For this review, take the finished solid that the model builds, in its own axes (mm). A direction names the side the tool comes from. Give positions to 0.01 mm unless a question says otherwise; leave off trailing zeros. Order: outer loops, then holes, each group sorted by start corner. A loop starts at its lowest first (then second) coordinate and runs counter-clockwise, first axis right, second up. Notation, with made-up numbers: (-9, 57.5) - (12, 57.5) arc R34 ccw to (12, 93.5) - close; hole circle Ø1 at (63, -13.5). An arc over 180 degrees is marked (long way). Answer as a JSON object with one key per item and string values. Group by question number.
from build123d import *

# Parameters (mm, degrees)
CYLINDER003_R     = 7
CYLINDER003_DEPTH = 4
CYLINDER002_R     = 5
CYLINDER002_DEPTH = 7
CYLINDER001_R     = 11
CYLINDER001_DEPTH = 3
CYLINDER_R        = 13
CYLINDER_DEPTH    = 4


with BuildPart() as cilindro003:
    # Cylinder003 → Cylinder003 (new body)
    with BuildSketch(Plane.XY.offset(3)):
        Circle(CYLINDER003_R)
    extrude(amount=CYLINDER003_DEPTH)


with BuildPart() as cilindro002:
    # Cylinder002 → Cylinder002 (new body)
    with BuildSketch(Plane.XY):
        Circle(CYLINDER002_R)
    extrude(amount=CYLINDER002_DEPTH)


with BuildPart() as cilindro001:
    # Cylinder001 → Cylinder001 (new body)
    with BuildSketch(Plane.XY.offset(4)):
        Circle(CYLINDER001_R)
    extrude(amount=CYLINDER001_DEPTH)


with BuildPart() as cut001:
    # Cylinder → Cylinder (new body)
    with BuildSketch(Plane.XY):
        Circle(CYLINDER_R)
    extrude(amount=CYLINDER_DEPTH)

    # Fusion: union Cilindro001
    add(cilindro001.part)

    # Cut: cut Cilindro002
    add(cilindro002.part, mode=Mode.SUBTRACT)

    # Cut001: cut Cilindro003
    add(cilindro003.part, mode=Mode.SUBTRACT)


solid = cut001.part
1) Mouldability with a two-part tool opening along X and no side actions: class faces 1 (the face through (6.466, -2.681, 4.972)), 2 (the face through (-11, 3, 4)), 3 (the face through (-10.316, -7.91, 1.972)) as released by +X, released by -X, zero draft, split by the parting line, or undercut.
2) Consider section A-A (y = 0). Give the boundary of the cut face in (x, z).
3) Consider section C-C (z = 3.5). Give the boundary of the cut face in (x, y), plus the area to 3 significant figures.
4) For pin 1 (1 mm diameter, centred on x = -10, z = 3.5, fed in from +Y); pin 2 (12 mm diameter, centred on x = -4.5, y = 9.5, fed in from -Z); pin 3 (4 mm diameter, centred on y = -4, z = 2.5, fed in from -X); pin 4 (4 mm diameter, centred on x = 7, z = 3.5, fed in from +Y), all flat-tipped, find the tip position at first contact; note any pin that passes through.
5) For faces 4 (the face through (-1.08, -4.88, 1.48)), 5 (the face through (-2.38, -10.74, 5.48)), list the 3-axis set-ups (+Z, -Z, +X, -X, +Y, -Y) from which the entire face can be reached by the end or side of a thin tool; tool diameter is ignored.
6) Consider section D-D (x = -6.5). Give the boundary of the cut face in (y, z), plus the area to 3 significant figures.
7) For line 1 (Y direction, x = 0, z = 4.55); line 2 (Y direction, x = 0, z = 1.2); line 3 (Z direction, x = -11.75, y = -4.25), list the stretches that pass through material, from the lowest coordinate up.
Result set:
{
 "1": {"face 1": "undercut", "face 2": "zero draft", "face 3": "split by the parting line"},
 "2": {"outline": "(-13, 0) - (-5, 0) - (-5, 3) - (-7, 3) - (-7, 7) - (-11, 7) - (-11, 4) - (-13, 4) - close; (5, 0) - (13, 0) - (13, 4) - (11, 4) - (11, 7) - (7, 7) - (7, 3) - (5, 3) - close"},
 "3": {"outline": "circle Ø26 at (0, 0); hole circle Ø14 at (0, 0)", "area": "377 mm2"},
 "4": {"pin 1": "stops at y = 8.87", "pin 2": "stops at z = 0", "pin 3": "stops at x = -12.85", "pin 4": "stops at y = 12"},
 "5": {"face 4": "+Z, -Z", "face 5": "+Z"},
 "6": {"outline": "(-11.26, 0) - (11.26, 0) - (11.26, 4) - (8.87, 4) - (8.87, 7) - (2.6, 7) - (2.6, 3) - (-2.6, 3) - (-2.6, 7) - (-8.87, 7) - (-8.87, 4) - (-11.26, 4) - close", "area": "123 mm2"},
 "7": {"line 1": "y = -11 to -7, 7 to 11", "line 2": "y = -13 to -5, 5 to 13", "line 3": "z = 0 to 4"}
}
